Design review of the part built by this model. Coordinates are the model's own, in mm. Face numbers are marked on the shaded views. A direction names the side the tool comes from. Round coordinates to 2 decimals unless told otherwise and drop trailing zeros. Write each loop counter-clockwise with the first axis right and the second up, starting at its lowest first coordinate (ties: lowest second). Pieces come first, ordered by that corner, then holes. Notation, with made-up numbers: M -21.5,20 L 15.5,20 A24 cw 15.5,54 Z; hole C -5.5,67 d6. An arc over 180 degrees is marked long. Use CSV: the item, a comma, the result in double quotes.
from build123d import *

# Parameters (mm, degrees)
SKETCH_1_R          = 19
SKETCH_1_R_2        = 17.6
EXTRUDE_1_DEPTH     = 3
SKETCH_2_R          = 19
EXTRUDE_2_DEPTH     = 4
SKETCH_3_R          = 1.6
SKETCH_3_R_2        = 2.1
CUT_EXTRUDE_1_DEPTH = 28.766886754


with BuildPart() as part:
    # 草图1 → 凸台-拉伸1 (new body)
    with BuildSketch(Plane(origin=(0, 0, 0), x_dir=(1, 0, 0), z_dir=(0, 1, 0))):
        with Locations(Location((0, 0, 0), (0, 0, 270))):
            Circle(SKETCH_1_R)
        with Locations(Location((0, 0, 0), (0, 0, 270))):
            Circle(SKETCH_1_R_2, mode=Mode.SUBTRACT)
    extrude(amount=EXTRUDE_1_DEPTH)

    # 草图2 → 凸台-拉伸2 (add)
    with BuildSketch(Plane(origin=(0, 3, 0), x_dir=(1, 0, 0), z_dir=(0, 1, 0))):
        with Locations(Location((0, 0, 0), (0, 0, 270))):
            Circle(SKETCH_2_R)
    extrude(amount=EXTRUDE_2_DEPTH)

    # 草图3 → 切除-拉伸1 (cut, through all)
    with BuildSketch(Plane(origin=(0, 7, 0), x_dir=(1, 0, 0), z_dir=(0, 1, 0))):
        with Locations(Location((0, 13.5, 0), (0, 0, 270))):
            Circle(SKETCH_3_R)
        with Locations(Location((11.691342951, 6.75, 0), (0, 0, 270))):
            Circle(SKETCH_3_R)
        with Locations(Location((11.691342951, -6.75, 0), (0, 0, 270))):
            Circle(SKETCH_3_R)
        with Locations(Location((0, -13.5, 0), (0, 0, 270))):
            Circle(SKETCH_3_R)
        with Locations(Location((-11.691342951, -6.75, 0), (0, 0, 270))):
            Circle(SKETCH_3_R)
        with Locations(Location((-11.691342951, 6.75, 0), (0, 0, 270))):
            Circle(SKETCH_3_R)
        with Locations(Location((12, 0, 0), (0, 0, 270))):
            Circle(SKETCH_3_R_2)
        with Locations(Location((-6, -10.392304845, 0), (0, 0, 270))):
            Circle(SKETCH_3_R_2)
        with Locations(Location((-6, 10.392304845, 0), (0, 0, 270))):
            Circle(SKETCH_3_R_2)
    extrude(amount=-CUT_EXTRUDE_1_DEPTH, mode=Mode.SUBTRACT)


solid = part.part
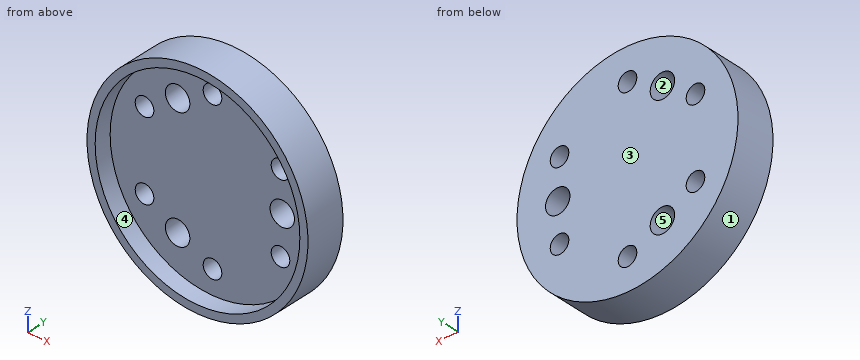
1) Machinability: for the marked faces 4 and 5, which of the approach directions +Z, -Z, +X, -X, +Y, -Y give a long, thin tool a straight path to every point of the face, cutting with its end or side? Answer none if there is none.
Answers:
face 4,"-Y"
face 5,"+Y, -Y"
2) Wall thickness on line 1 along X through (y, z) = (4.35, 6.75); line 2 along X through (y, z) = (5.15, 0); line 3 along Y through (x, z) = (14, -2.5): over which ranges is each line inside the solid? List them lowest first. Write a range as [from, to].
Answers:
line 1,"[-17.76, -13.29], [-10.09, 10.09], [13.29, 17.76]"
line 2,"[-19, 9.9], [14.1, 19]"
line 3,"[3, 7]"
3) For pin 1 Ø5 at (x, z) = (11.69, 6.75) entering from +Y; pin 2 Ø4 at (y, z) = (1.5, 1.5) entering from +X; pin 3 Ø3 at (y, z) = (5.5, 6.5) entering from -X; pin 4 Ø4 at (x, z) = (7, 9) entering from -Y, all flat-tipped, find the tip position at first contact; note any pin that passes through.
Answers:
pin 1,"y = 7"
pin 2,"x = 19"
pin 3,"x = -18.33"
pin 4,"y = 3"
4) Add section C-C on z = -6.75. Write out the cut boundary in (x, y).
Answers:
outline,"M -17.76,0 L -16.25,0 L -16.25,3 L -13.29,3 L -13.29,7 L -17.76,7 Z; M -10.09,3 L 10.09,3 L 10.09,7 L -10.09,7 Z; M 13.29,3 L 16.25,3 L 16.25,0 L 17.76,0 L 17.76,7 L 13.29,7 Z"
5) Add section D-D on y = 2.5. Write out the cut boundary in (x, z), then the cut area to 3 significant figures.
Answers:
outline,"C 0,0 d38; hole C 0,0 d35.2"
area,"161 mm²"
6) The part is to be moulded in two halves that separate along Z. For the marked faces 1, 2 and 3, say which applies: released by +Z, released by -Z, zero draft, split by the parting line, or undercut.
Answers:
face 1,"split by the parting line"
face 2,"undercut"
face 3,"zero draft"
7) Add section A-A on z = 0. Write out the cut boundary in (x, y).
Answers:
outline,"M -19,0 L -17.6,0 L -17.6,3 L 9.9,3 L 9.9,7 L -19,7 Z; M 14.1,3 L 17.6,3 L 17.6,0 L 19,0 L 19,7 L 14.1,7 Z"
8) Add section B-B on x = -6. Write out the cut boundary in (y, z), then the cut area to 3 significant figures.
Answers:
outline,"M 0,-18.03 L 7,-18.03 L 7,-12.49 L 3,-12.49 L 3,-16.55 L 0,-16.55 Z; M 0,16.55 L 3,16.55 L 3,12.49 L 7,12.49 L 7,18.03 L 0,18.03 Z; M 3,-8.29 L 7,-8.29 L 7,8.29 L 3,8.29 Z"
area,"120 mm²"
